Part print with two shaded views. Sizes in mm from the minimum x, y, z corner. Coordinates: 2 decimals unless noted, no trailing zeros. Write each loop counter-clockwise with the first axis right and the second up, starting at its lowest first coordinate (ties: lowest second). Pieces come first, ordered by that corner, then holes.
Q1. Pin check, flat tip, straight feed: P1, Ø1.5, axis at y = 6, z = 16.5, coming from the -X side. Stop position of the tip, or through.
Q2. Band-saw the part on A-A, the plane x = 68. Write the cut outline in (y, z).
Q3. Band-saw the part on D-D, the plane y = 3. Write the cut outline in (x, z).
Q4. Pull direction X, two halves, no side cores. Call the marked faces 1, 2 and 3: released by +X, released by -X, zero draft, split by the parting line, or undercut.
Q5. Band-saw the part on B-B, the plane z = 10. Write the cut outline in (x, y).
Q6. Drill centre lines: probe 1 along Z at (x, y) = (10, 5); probe 2 along X at (y, z) = (7.75, 15.25); probe 3 along X at (y, z) = (7, 16). Where is each one in solid material? Low to high.
Q7. Band-saw the part on C-C, the plane y = 7. Write the cut outline in (x, z).
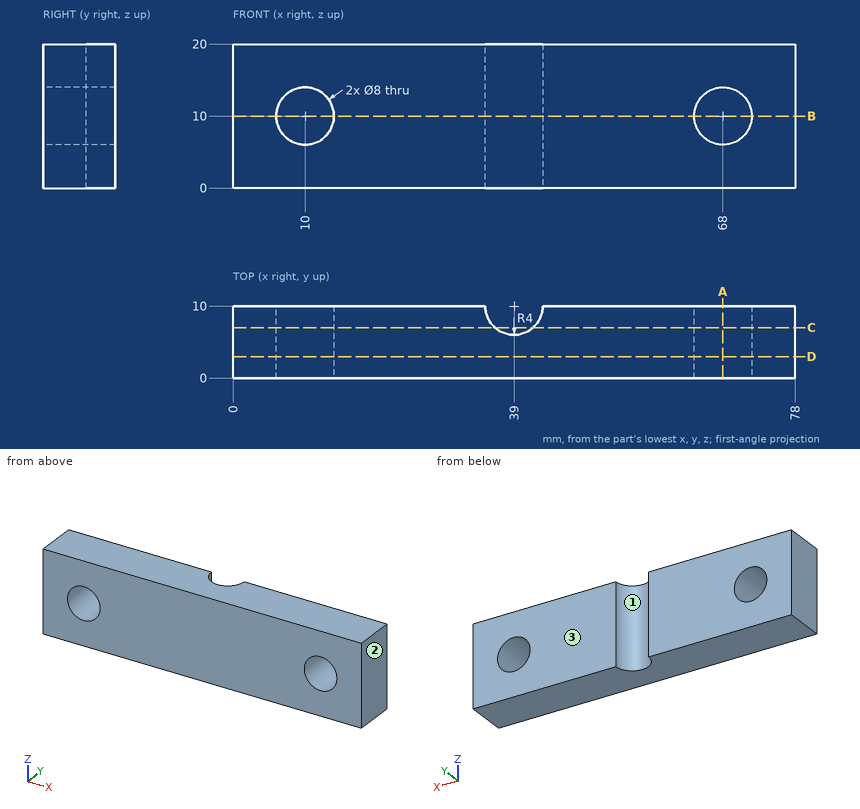
Answer sheet:
1. P1: stops at x = 0
2. outline: (0, 0) - (10, 0) - (10, 6) - (0, 6) - close; (0, 14) - (10, 14) - (10, 20) - (0, 20) - close
3. outline: (0, 0) - (78, 0) - (78, 20) - (0, 20) - close; hole circle Ø8 at (10, 10); hole circle Ø8 at (68, 10)
4. face 1: undercut
4. face 2: released by +X
4. face 3: zero draft
5. outline: (0, 0) - (6, 0) - (6, 10) - (0, 10) - close; (14, 0) - (64, 0) - (64, 10) - (43, 10) arc R4 cw to (35, 10) - (14, 10) - close; (72, 0) - (78, 0) - (78, 10) - (72, 10) - close
6. probe 1: z = 0 to 6, 14 to 20
6. probe 2: x = 0 to 35.69, 42.31 to 78
6. probe 3: x = 0 to 36.35, 41.65 to 78
7. outline: (0, 0) - (36.35, 0) - (36.35, 20) - (0, 20) - close; (41.65, 0) - (78, 0) - (78, 20) - (41.65, 20) - close; hole circle Ø8 at (10, 10); hole circle Ø8 at (68, 10)
